Verification items for the finished model (mm, model axes). A direction names the side the tool comes from. Coordinates: 2 decimals unless noted, no trailing zeros. Order: outer loops, then holes, each group sorted by start corner. A loop starts at its lowest first (then second) coordinate and runs counter-clockwise, first axis right, second up. Notation, with made-up numbers: M 68,-37 L 127,-37 A18 cw 127,-27 Z; hole C 84.25,63 d11. An arc over 180 degrees is marked long. Return JSON: item names as keys, results as strings. Group by question number.
1. Section check B-B, the plane y = 4.5. Record the cut outline in (x, z).
2. Material ranges on line 1 along X through (y, z) = (33.75, 5); line 2 along Y through (x, z) = (18.5, 5); line 3 along Z through (x, y) = (-10.2, 35), recorded low to high.
3. Set-up check for faces 1 (the flat face through (33.491, -33.59, -12.035)), 2 (the cylindrical face through (-17.88, -0.07, 3.35)), 3 (the flat face through (-21.6, -36.6, 3.7)): record each of +Z, -Z, +X, -X, +Y, -Y from which the full face is reachable in a straight line by a thin tool's end or side.
4. Gauge pin test, flat ends, axial feed: pin 1 (2 mm diameter, centred on x = -10.2, z = 5, fed in from -Y); pin 2 (4.5 mm diameter, centred on y = -16.5, z = 5.5, fed in from -X); pin 3 (1.6 mm diameter, centred on y = 12, z = -3, fed in from -X); pin 4 (5.5 mm diameter, centred on x = 10.2, z = 5, fed in from -Y). Record the tip position at first contact, or that the pin passes through.
5. Section check D-D, the plane x = 18. Record the cut outline in (y, z).
6. Section check A-A, the plane z = 1.75. Record the cut outline in (x, y).
7. Mould release check, pull along Z, two halves, no side actions. Record for faces 4 (the flat face through (-21.6, 36.6, 3.6)), 5 (the flat face through (21.232, -36.271, 9.122)), 6 (the cylindrical face through (-9.085, -32.879, 3.784)): +Z half, -Z half, draft (parallel to the pull), parting line (faces both ways), or undercut.
8. Section check C-C, the plane z = -3. Record the cut outline in (x, y).
```python
from build123d import *

# Parameters (mm, degrees)
BOSS_EXTRUDE1_DEPTH             = 38
BOSS_EXTRUDE1_DEPTH_BACK        = 38
SKETCH2_W                       = 46
SKETCH2_H                       = 76
BOSS_EXTRUDE2_DEPTH             = 10
ADVANCEDHOLE1_START             = 9.350877343
ADVANCEDHOLE1_OUTLINE_R         = 5.5
ADVANCEDHOLE1_DEPTH             = 2.175616923
ADVANCEDHOLE1_START_2           = 5.350877343
ADVANCEDHOLE1_2_OUTLINE_R       = 3.2
ADVANCEDHOLE1_2_DEPTH           = 4
ADVANCEDHOLE2_START             = -11.526494266
ADVANCEDHOLE2_OUTLINE_R         = 5.5
ADVANCEDHOLE2_DEPTH             = 2.175616923
ADVANCEDHOLE2_START_2           = -9.350877343
ADVANCEDHOLE2_2_OUTLINE_R       = 3.2
ADVANCEDHOLE2_2_DEPTH           = 4
SKETCH11_W                      = 2
SKETCH11_H                      = 76
CUT_EXTRUDE1_DEPTH              = 1
M4_TAPPED_HOLE1_D               = 3.3
M4_TAPPED_HOLE1_DEPTH           = 10.1
M4_TAPPED_HOLE1_TIP             = 0.991420021
M4_TAPPED_HOLE1_ON_FACE_2_D     = 3.3
M4_TAPPED_HOLE1_ON_FACE_2_DEPTH = 10.1
M4_TAPPED_HOLE1_ON_FACE_2_TIP   = 0.991420021
M4_TAPPED_HOLE1_ON_FACE_3_D     = 3.3
M4_TAPPED_HOLE1_ON_FACE_3_DEPTH = 10.1
M4_TAPPED_HOLE1_ON_FACE_3_TIP   = 0.991420021
M4_TAPPED_HOLE1_ON_FACE_4_D     = 3.3
M4_TAPPED_HOLE1_ON_FACE_4_DEPTH = 10.1
M4_TAPPED_HOLE1_ON_FACE_4_TIP   = 0.991420021
CHAMFER1_SIZE                   = 2.8
CHAMFER2_SIZE                   = 1
CHAMFER2_SIZE2                  = 1.732050808


# Read off the part's stored shape, not the designer's step: AdvancedHole1, AdvancedHole2
with BuildPart() as part:
    # Sketch1 → Boss-Extrude1 (new, two sides: drawn at the far end of the back side and taken through both)
    with BuildSketch(Plane(origin=(0, 0, 0), x_dir=(1, 0, 0), z_dir=(0, 1, 0)).offset(-BOSS_EXTRUDE1_DEPTH_BACK)):
        Polygon((-25, 2), (-40.107437881, 16.6682169), (-37.813132135, 19.944825077), (-15, 3.970897986), (-15, 2), (15, 2), (15, 3.970897986), (37.813132135, 19.944825077), (40.107437881, 16.6682169), (25, 2), (25, 0), (-25, 0), align=None)
    extrude(amount=BOSS_EXTRUDE1_DEPTH + BOSS_EXTRUDE1_DEPTH_BACK)

    # Sketch2 → Boss-Extrude2 (add)
    with BuildSketch(Plane.XY):
        Rectangle(SKETCH2_W, SKETCH2_H)
    extrude(amount=BOSS_EXTRUDE2_DEPTH)

    # AdvancedHole1 outline → AdvancedHole1 (cut)
    with BuildSketch(Plane(origin=(0, 0, 0), x_dir=(0.819152044288991, 0, -0.5735764363510472), z_dir=(0.5735764363510472, 0, 0.8191520442889911)).offset(ADVANCEDHOLE1_START)):
        with Locations((34.414586181, -30)):
            Circle(ADVANCEDHOLE1_OUTLINE_R)
        with Locations((34.414586181, 15)):
            Circle(ADVANCEDHOLE1_OUTLINE_R)
    extrude(amount=ADVANCEDHOLE1_DEPTH, mode=Mode.SUBTRACT)

    # AdvancedHole1 2 outline → AdvancedHole1 2 (cut)
    with BuildSketch(Plane(origin=(0, 0, 0), x_dir=(0.819152044288991, 0, -0.5735764363510472), z_dir=(0.5735764363510472, 0, 0.8191520442889911)).offset(ADVANCEDHOLE1_START_2)):
        with Locations((34.414586181, -30)):
            Circle(ADVANCEDHOLE1_2_OUTLINE_R)
        with Locations((34.414586181, 15)):
            Circle(ADVANCEDHOLE1_2_OUTLINE_R)
    extrude(amount=ADVANCEDHOLE1_2_DEPTH, mode=Mode.SUBTRACT)

    # AdvancedHole2 outline → AdvancedHole2 (cut)
    with BuildSketch(Plane(origin=(0, 0, 0), x_dir=(0.819152044288991, 0, 0.5735764363510472), z_dir=(0.5735764363510472, 0, -0.8191520442889911)).offset(ADVANCEDHOLE2_START)):
        with Locations((-34.414586181, 30)):
            Circle(ADVANCEDHOLE2_OUTLINE_R)
        with Locations((-34.414586181, -15)):
            Circle(ADVANCEDHOLE2_OUTLINE_R)
    extrude(amount=ADVANCEDHOLE2_DEPTH, mode=Mode.SUBTRACT)

    # AdvancedHole2 2 outline → AdvancedHole2 2 (cut)
    with BuildSketch(Plane(origin=(0, 0, 0), x_dir=(0.819152044288991, 0, 0.5735764363510472), z_dir=(0.5735764363510472, 0, -0.8191520442889911)).offset(ADVANCEDHOLE2_START_2)):
        with Locations((-34.414586181, 30)):
            Circle(ADVANCEDHOLE2_2_OUTLINE_R)
        with Locations((-34.414586181, -15)):
            Circle(ADVANCEDHOLE2_2_OUTLINE_R)
    extrude(amount=ADVANCEDHOLE2_2_DEPTH, mode=Mode.SUBTRACT)

    # Sketch11 → Cut-Extrude1 (cut)
    with BuildSketch(Plane.XY):
        with Locations((-24, 0)):
            Rectangle(SKETCH11_W, SKETCH11_H)
    extrude(amount=-CUT_EXTRUDE1_DEPTH, mode=Mode.SUBTRACT)

    # M4 Tapped Hole1
    with Locations(Plane(origin=(23, 30, 5), x_dir=(0, 1, 0), z_dir=(1, 0, 0))):
        with Locations((0, 0), (-60, 0), (-30, 0)):
            Hole(M4_TAPPED_HOLE1_D / 2, depth=M4_TAPPED_HOLE1_DEPTH)
            with Locations((0, 0, -(M4_TAPPED_HOLE1_DEPTH + M4_TAPPED_HOLE1_TIP / 2))):  # 118° drill point
                Cone(0, M4_TAPPED_HOLE1_D / 2, M4_TAPPED_HOLE1_TIP, mode=Mode.SUBTRACT)

    # M4 Tapped Hole1 on face 2
    with Locations(Plane(origin=(-23, 30, 5), x_dir=(0, 0, -1), z_dir=(-1, 0, 0))):
        with Locations((0, 0), (0, 60), (0, 30)):
            Hole(M4_TAPPED_HOLE1_ON_FACE_2_D / 2, depth=M4_TAPPED_HOLE1_ON_FACE_2_DEPTH)
            with Locations((0, 0, -(M4_TAPPED_HOLE1_ON_FACE_2_DEPTH + M4_TAPPED_HOLE1_ON_FACE_2_TIP / 2))):  # 118° drill point
                Cone(0, M4_TAPPED_HOLE1_ON_FACE_2_D / 2, M4_TAPPED_HOLE1_ON_FACE_2_TIP, mode=Mode.SUBTRACT)

    # M4 Tapped Hole1 on face 3
    with Locations(Plane(origin=(10.2, 38, 5), x_dir=(0, 0, 1), z_dir=(0, 1, 0))):
        with Locations((0, 0), (0, -20.4)):
            Hole(M4_TAPPED_HOLE1_ON_FACE_3_D / 2, depth=M4_TAPPED_HOLE1_ON_FACE_3_DEPTH)
            with Locations((0, 0, -(M4_TAPPED_HOLE1_ON_FACE_3_DEPTH + M4_TAPPED_HOLE1_ON_FACE_3_TIP / 2))):  # 118° drill point
                Cone(0, M4_TAPPED_HOLE1_ON_FACE_3_D / 2, M4_TAPPED_HOLE1_ON_FACE_3_TIP, mode=Mode.SUBTRACT)

    # M4 Tapped Hole1 on face 4
    with Locations(Plane(origin=(-10.2, -38, 5), x_dir=(0, 0, -1), z_dir=(0, -1, 0))):
        with Locations((0, 0), (0, 20.4)):
            Hole(M4_TAPPED_HOLE1_ON_FACE_4_D / 2, depth=M4_TAPPED_HOLE1_ON_FACE_4_DEPTH)
            with Locations((0, 0, -(M4_TAPPED_HOLE1_ON_FACE_4_DEPTH + M4_TAPPED_HOLE1_ON_FACE_4_TIP / 2))):  # 118° drill point
                Cone(0, M4_TAPPED_HOLE1_ON_FACE_4_D / 2, M4_TAPPED_HOLE1_ON_FACE_4_TIP, mode=Mode.SUBTRACT)

    # Chamfer1
    chamfer1_edges = [part.edges().sort_by_distance(p)[0] for p in [
        (23, -38, 5),
        (23, 38, 5),
        (-23, 38, 4.5),
        (-23, -38, 4.5),
    ]]
    chamfer(chamfer1_edges, length=CHAMFER1_SIZE)

    # Chamfer2
    chamfer2_edges = [part.edges().sort_by_distance(p)[0] for p in [
        (23, 0, 10),
        (0, -38, 10),
        (0, 38, 10),
        (-23, 0, 10),
        (21.6, 36.6, 10),
        (-21.6, 36.6, 10),
        (-21.6, -36.6, 10),
        (21.6, -36.6, 10),
    ]]
    chamfer2_side = [part.faces().sort_by_distance(p)[0] for p in [
        (0, 0, 10),
    ]]
    chamfer(chamfer2_edges, length=CHAMFER2_SIZE, length2=CHAMFER2_SIZE2, reference=chamfer2_side[0])


solid = part.part
```
Answers follow:
{
 "1": {"outline": "M -40.11,-16.67 L -37.81,-19.94 L -15,-3.97 L -15,-2 L 15,-2 L 15,-3.97 L 37.81,-19.94 L 40.11,-16.67 L 25,-2 L 25,0 L 23,0 L 23,8.27 L 22,10 L -22,10 L -23,8.27 L -23,-1 L -25,-1 L -25,-2 Z"},
 "2": {"line 1": "-23 to -11.85, -8.55 to 8.55, 11.85 to 23", "line 2": "-38 to -31.65, -28.35 to -1.65, 1.65 to 28.35, 31.65 to 38", "line 3": "-2 to 3.35, 6.65 to 10"},
 "3": {"face 1": "none", "face 2": "-X", "face 3": "+Z, -X, -Y"},
 "4": {"pin 1": "y = -27.51", "pin 2": "x = -23", "pin 3": "x = -26.85", "pin 4": "y = -38"},
 "5": {"outline": "M -38,-6.07 L 38,-6.07 L 38,8.27 L 37,10 L -37,10 L -38,8.27 Z; hole C -30,5 d3.3; hole C 0,5 d3.3; hole C 30,5 d3.3"},
 "6": {"outline": "M -23,-35.2 L -20.2,-38 L 20.2,-38 L 23,-35.2 L 23,35.2 L 20.2,38 L -20.2,38 L -23,35.2 Z"},
 "7": {"face 4": "draft", "face 5": "+Z half", "face 6": "undercut"},
 "8": {"outline": "M -26.03,-38 L -15,-38 L -15,38 L -26.03,38 Z; M 15,-38 L 26.03,-38 L 26.03,38 L 15,38 Z"}
}
